Here's how the part is built. I have some questions about the finished solid (model axes, mm). A direction names the side the tool comes from. Round coordinates to 2 decimals unless told otherwise and drop trailing zeros. Loops run counter-clockwise (first coordinate to the right, second up) from the corner with the lowest first, then second, coordinate; pieces in that order, holes last. Notation, with made-up numbers: M 17.5,-29.5 L 76.5,-29.5 A20 ccw 76.5,-11.5 Z; hole C 10,33 d5. An arc over 180 degrees is marked long. Use a Markdown table: item, result.
from build123d import *

# Parameters (mm, degrees)
SKETCH1_R           = 25
BOSS_EXTRUDE1_DEPTH = 150
SKETCH2_R           = 42.5
BOSS_EXTRUDE2_DEPTH = 30
FILLET4_R           = 8
FILLET5_R           = 8
SKETCH4_R           = 1.6
CUT_EXTRUDE1_DEPTH  = 30
CUT_EXTRUDE4_DEPTH  = 155
SKETCH6_R           = 10
CUT_EXTRUDE5_DEPTH  = 8


with BuildPart() as part:
    # Sketch1 → Boss-Extrude1 (new body)
    with BuildSketch(Plane.XY):
        Circle(SKETCH1_R)
    extrude(amount=BOSS_EXTRUDE1_DEPTH)

    # Sketch2 → Boss-Extrude2 (add)
    with BuildSketch(Plane.XY):
        Circle(SKETCH2_R)
    extrude(amount=-BOSS_EXTRUDE2_DEPTH)

    # Sketch3 → Revolve1 (revolve)
    with BuildSketch(Plane(origin=(0, 0, 0), x_dir=(1, 0, 0), z_dir=(0, 1, 0))):
        Polygon((25, 0), (25, -15), (42.5, 0), align=None)
    revolve(axis=Axis((0, 0, 0), (0, 0, 1)))

    # Fillet4
    fillet4_edges = [part.edges().sort_by_distance(p)[0] for p in [
        (-25, 0, 15),
    ]]
    fillet(fillet4_edges, radius=FILLET4_R)

    # Fillet5
    fillet5_edges = [part.edges().sort_by_distance(p)[0] for p in [
        (-42.5, 0, 0),
    ]]
    fillet(fillet5_edges, radius=FILLET5_R)

    # Sketch4 → Cut-Extrude1 (cut)
    with BuildSketch(Plane.XY):
        Circle(SKETCH4_R)
        with Locations((-10, 0)):
            Circle(SKETCH4_R)
        with Locations((10, 0)):
            Circle(SKETCH4_R)
    extrude(amount=-CUT_EXTRUDE1_DEPTH, mode=Mode.SUBTRACT)

    # Sketch5 → Cut-Extrude4 (cut)
    with BuildSketch(Plane.XY.offset(150)):
        Polygon((-7.61843014, -1.375), (-7.61843014, 1.375), (-10, 2.75), (-12.38156986, 1.375), (-12.38156986, -1.375), (-10, -2.75), align=None)
        Polygon((0, -2.75), (2.38156986, -1.375), (2.38156986, 1.375), (0, 2.75), (-2.38156986, 1.375), (-2.38156986, -1.375), align=None)
        Polygon((10, -2.75), (12.38156986, -1.375), (12.38156986, 1.375), (10, 2.75), (7.61843014, 1.375), (7.61843014, -1.375), align=None)
    extrude(amount=-CUT_EXTRUDE4_DEPTH, mode=Mode.SUBTRACT)

    # Sketch6 → Cut-Extrude5 (cut)
    with BuildSketch(Plane(origin=(0, 0, -30), x_dir=(-1, 0, 0), z_dir=(0, 0, -1))):
        with Locations((30, 0)):
            Circle(SKETCH6_R)
        with Locations((-30, 0)):
            Circle(SKETCH6_R)
    extrude(amount=-CUT_EXTRUDE5_DEPTH, mode=Mode.SUBTRACT)


solid = part.part
1. Imagine slicing it at B-B, the plane z = -12.5. Write out the boundary of the cut face in (x, y), then the cut area to 3 significant figures.
Answer sheet:
| item | result |
|---|---|
| outline | C 0,0 d85; hole C -10,0 d3.2; hole C 0,0 d3.2; hole C 10,0 d3.2 |
| area | 5,650 mm2 |
2. We'd pull the mould along X, two halves only. Please class faces 1 (the face through (-30, 0, -22)), 2 (the face through (8, 0, -5)), 3 (the face through (27.22, 8.57, 11.97)), 4 (the face through (-1, -9, -30)): +X half, -X half, draft (parallel to the pull), parting line (faces both ways), or undercut.
Answer sheet:
| item | result |
|---|---|
| face 1 | undercut |
| face 2 | undercut |
| face 3 | parting line |
| face 4 | draft |
3. Which directions (+Z, -Z, +X, -X, +Y, -Y) give clear straight access to the entire face, cutting with the end or side of a thin tool? Please do faces 5 (the face through (-12, 0, -5)), 6 (the face through (-39.54, 3, -26.06)), 7 (the face through (0, -5, 150)).
Answer sheet:
| item | result |
|---|---|
| face 5 | +Z |
| face 6 | -Z |
| face 7 | +Z, +X, -X, +Y, -Y |
4. I need wall thicknesses on probe 1 along X at (y, z) = (-2, 3); probe 2 along Z at (x, y) = (23, 7); probe 3 along Y at (x, z) = (12, 126). Which ranges of each line are inside material? Lowest first, please. Write a range as from..to.
Answer sheet:
| item | result |
|---|---|
| probe 1 | -38.95..-11.3, -8.7..-1.3, 1.3..8.7, 11.3..38.95 |
| probe 2 | -22..150 |
| probe 3 | -21.93..-1.6, 1.6..21.93 |
5. For pin 1 Ø4 at (x, y) = (29.5, 25) entering from +Z; pin 2 Ø2 at (y, z) = (-0.5, 85.5) entering from -X; pin 3 Ø4 at (x, y) = (3, 33.5) entering from +Z; pin 4 Ø1.9 at (x, y) = (0, 0) entering from +Z, each with a flat end and sliding along its axis, tell me the tip position at first contact or that it passes through.
Answer sheet:
| item | result |
|---|---|
| pin 1 | z = 5 |
| pin 2 | x = -25 |
| pin 3 | z = 9.31 |
| pin 4 | through |
6. Imagine slicing it at A-A, the plane z = 58. Write out the boundary of the cut face in (x, y) (3 decimals).
Answer sheet:
| item | result |
|---|---|
| outline | C 0,0 d50; hole M -12.382,-1.375 L -10,-2.75 L -7.618,-1.375 L -7.618,1.375 L -10,2.75 L -12.382,1.375 Z; hole M -2.382,-1.375 L 0,-2.75 L 2.382,-1.375 L 2.382,1.375 L 0,2.75 L -2.382,1.375 Z; hole M 7.618,-1.375 L 10,-2.75 L 12.382,-1.375 L 12.382,1.375 L 10,2.75 L 7.618,1.375 Z |
